```python
from build123d import *

# Parameters (mm, degrees)
SKETCH_1_W          = 70
SKETCH_1_H          = 75
SKETCH_1_R          = 12.5
SKETCH_1_R_2        = 1.75
EXTRUDE_1_DEPTH     = 10
EXTRUDE_3_DEPTH     = 5
EXTRUDE_4_DEPTH     = 5
SKETCH_7_W          = 70
SKETCH_7_H          = 180
EXTRUDE_5_DEPTH     = 5
SKETCH_10_R         = 1.8
CUT_EXTRUDE_2_DEPTH = 197.277864264
SKETCH_11_R         = 1.75
CUT_EXTRUDE_3_DEPTH = 199.305320151


with BuildPart() as part:
    # 草图1 → 凸台-拉伸1 (new body)
    with BuildSketch(Plane(origin=(0, 0, 0), x_dir=(1, 0, 0), z_dir=(0, 1, 0))):
        with Locations((0, -7.5)):
            Rectangle(SKETCH_1_W, SKETCH_1_H)
        with Locations(Location((0, 0, 0), (0, 0, 270))):
            Circle(SKETCH_1_R, mode=Mode.SUBTRACT)
        with Locations(Location((0, 20, 0), (0, 0, 270))):
            Circle(SKETCH_1_R_2, mode=Mode.SUBTRACT)
        with Locations(Location((17.320508076, -10, 0), (0, 0, 270))):
            Circle(SKETCH_1_R_2, mode=Mode.SUBTRACT)
        with Locations(Location((-17.320508076, -10, 0), (0, 0, 270))):
            Circle(SKETCH_1_R_2, mode=Mode.SUBTRACT)
    extrude(amount=EXTRUDE_1_DEPTH)

    # 草图6 → 凸台-拉伸3 (add)
    with BuildSketch(Plane.ZY.offset(35)):
        Polygon((40, 180), (-30, 25), (-30, 0), (45, 0), (45, 180), align=None)
    extrude(amount=-EXTRUDE_3_DEPTH)

    # 草图8 → 凸台-拉伸4 (add)
    with BuildSketch(Plane(origin=(35, 0, 0), x_dir=(0, 0, -1), z_dir=(1, 0, 0))):
        Polygon((-45, 0), (-45, 180), (-40, 180), (30, 25), (30, 0), align=None)
    extrude(amount=-EXTRUDE_4_DEPTH)

    # 草图7 → 凸台-拉伸5 (add)
    with BuildSketch(Plane.XY.offset(45)):
        with Locations((0, 90)):
            Rectangle(SKETCH_7_W, SKETCH_7_H)
    extrude(amount=-EXTRUDE_5_DEPTH)

    # 草图10 → 切除-拉伸2 (cut, through all)
    with BuildSketch(Plane(origin=(0, 0, 40), x_dir=(-1, 0, 0), z_dir=(0, 0, -1))):
        with Locations((-23.375, 171)):
            Circle(SKETCH_10_R)
        with Locations((23.375, 171)):
            Circle(SKETCH_10_R)
        with Locations((0, 171)):
            Circle(SKETCH_10_R)
    extrude(amount=-CUT_EXTRUDE_2_DEPTH, mode=Mode.SUBTRACT)

    # 草图11 → 切除-拉伸3 (cut, through all)
    with BuildSketch(Plane.ZY.offset(35)):
        with Locations((35, 132.484247104)):
            Circle(SKETCH_11_R)
        with Locations((35, 15)):
            Circle(SKETCH_11_R)
        with Locations((-20, 15)):
            Circle(SKETCH_11_R)
        with BuildLine():
            Line((35, 102.837189188), (35, 29))
            ThreePointArc((35, 29), (32.363961031, 22.636038969), (26, 20))
            Line((26, 20), (-7.345827375, 20))
            ThreePointArc((-7.345827375, 20), (-14.906863168, 24.118326338), (-15.548162772, 32.704280502))
            Line((-15.548162772, 32.704280502), (17.797664603, 106.54146969))
            ThreePointArc((17.797664603, 106.54146969), (27.894595132, 111.63551342), (35, 102.837189188))
        make_face()
    extrude(amount=-CUT_EXTRUDE_3_DEPTH, mode=Mode.SUBTRACT)


solid = part.part
```
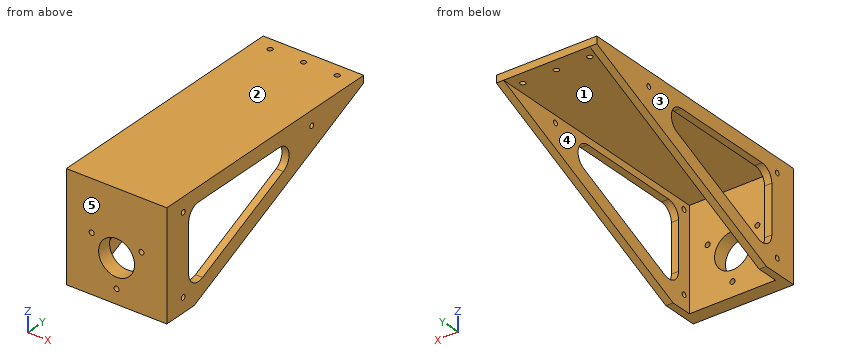
Read the model definition and answer for the solid it produces. Units are mm, in the model's axes. Face numbers are marked on the shaded views. A direction names the side the tool comes from. Coordinates: 2 decimals unless noted, no trailing zeros. Loops run counter-clockwise (first coordinate to the right, second up) from the corner with the lowest first, then second, coordinate; pieces in that order, holes last.
(1) Consider line 1 along X through (y, z) = (47, 37.5); line 2 along X through (y, z) = (6, 0); line 3 along Z through (x, y) = (-22.5, 90). Determine where each line is inside the solid, lowest interval first.
Solution:
line 1: x = -35 to -30, 30 to 35
line 2: x = -35 to -12.5, 12.5 to 35
line 3: z = 40 to 45
(2) The part is cut by section C-C (z = -20). Determine the outline of the cut face in (x, y).
Solution:
outline: (-35, 0) - (-1.75, 0) - (-1.75, 10) - (-30, 10) - (-30, 13.25) - (-35, 13.25) - close; (-35, 16.75) - (-30, 16.75) - (-30, 47.14) - (-35, 47.14) - close; (1.75, 0) - (35, 0) - (35, 13.25) - (30, 13.25) - (30, 10) - (1.75, 10) - close; (30, 16.75) - (35, 16.75) - (35, 47.14) - (30, 47.14) - close
(3) The part is cut by section A-A (x = 0). Determine the outline of the cut face in (y, z), and give its area (3 significant figures).
Solution:
outline: (0, -30) - (10, -30) - (10, -21.75) - (0, -21.75) - close; (0, -18.25) - (10, -18.25) - (10, -12.5) - (0, -12.5) - close; (0, 12.5) - (10, 12.5) - (10, 40) - (169.2, 40) - (169.2, 45) - (0, 45) - close; (172.8, 40) - (180, 40) - (180, 45) - (172.8, 45) - close
area: 1,300 mm2
(4) A tool of negligible diameter and unlimited length cuts with its end or side. For the marked faces 1 and 2, from which of +Z, -Z, +X, -X, +Y, -Y can it reach the whole face along a straight path? Write none if from no direction.
Solution:
face 1: -Z, +Y
face 2: +Z, +X, -X, +Y, -Y
(5) Flat-ended cylindrical pins translate along their axes: pin 1 Ø5 at (x, y) = (3.5, 24) entering from -Z; pin 2 Ø22.5 at (x, z) = (0, 0) entering from +Y; pin 3 Ø2.5 at (x, y) = (32, 57) entering from -Z; pin 4 Ø4 at (x, z) = (-32, 9) entering from +Y. Find the tip coordinate at first contact, or state that the pin passes through.
Solution:
pin 1: stops at z = 40
pin 2: passes through
pin 3: stops at z = -16.11
pin 4: stops at y = 115.79
(6) The part is cut by section B-B (y = 15). Determine the outline of the cut face in (x, z).
Solution:
outline: (-35, -30) - (-30, -30) - (-30, -21.75) - (-35, -21.75) - close; (-35, -18.25) - (-30, -18.25) - (-30, 33.25) - (-35, 33.25) - close; (-35, 36.75) - (-30, 36.75) - (-30, 40) - (30, 40) - (30, 36.75) - (35, 36.75) - (35, 45) - (-35, 45) - close; (30, -30) - (35, -30) - (35, -21.75) - (30, -21.75) - close; (30, -18.25) - (35, -18.25) - (35, 33.25) - (30, 33.25) - close
(7) The mould has two halves that part along X. Classify the marked faces 3, 4 and 5: released by +X, released by -X, zero draft, split by the parting line, or undercut.
Solution:
face 3: released by -X
face 4: undercut
face 5: zero draft
(8) The part is cut by section D-D (y = 98.5). Determine the outline of the cut face in (x, z).
Solution:
outline: (-35, 3.19) - (-30, 3.19) - (-30, 14.17) - (-35, 14.17) - close; (-35, 35) - (-30, 35) - (-30, 40) - (30, 40) - (30, 35) - (35, 35) - (35, 45) - (-35, 45) - close; (30, 3.19) - (35, 3.19) - (35, 14.17) - (30, 14.17) - close
